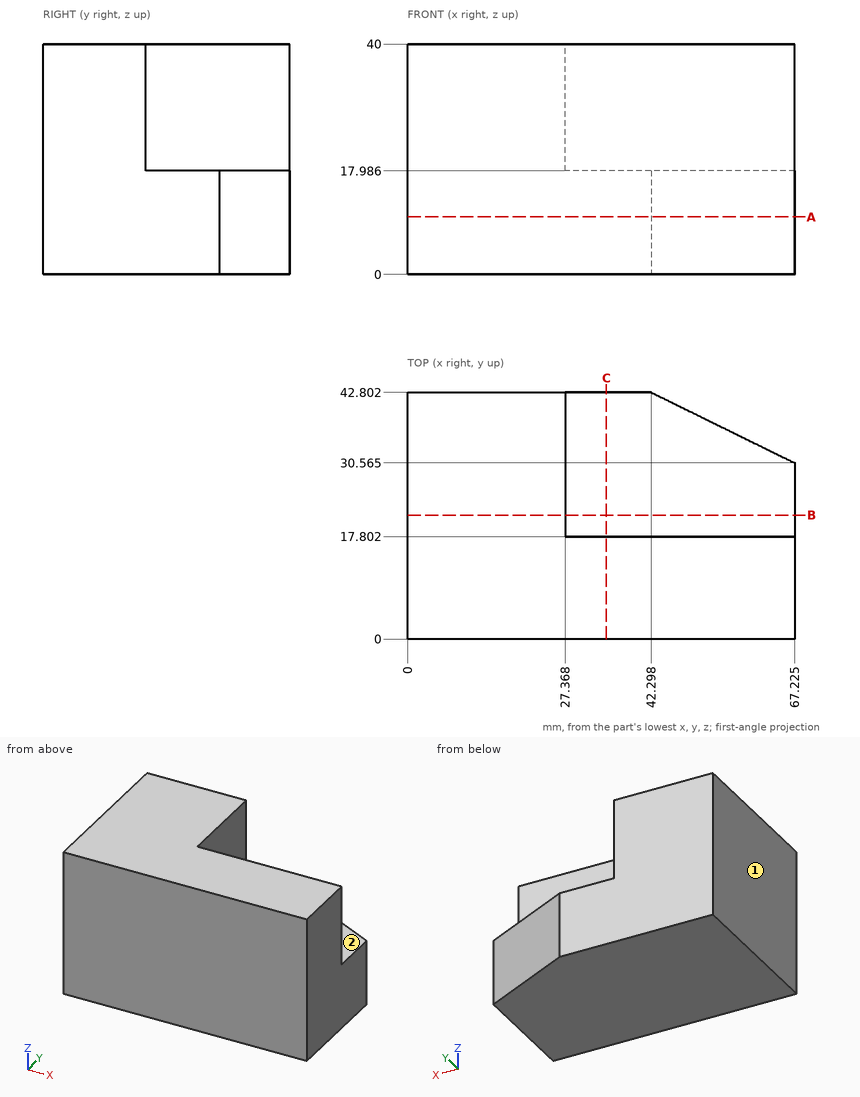
Geometry check sheet. Reference: drawing and pictorial views, mm from the part's lowest x, y, z. A direction names the side the tool comes from. Coordinates: 2 decimals unless noted, no trailing zeros. Order: outer loops, then holes, each group sorted by start corner. A loop starts at its lowest first (then second) coordinate and runs counter-clockwise, first axis right, second up.
1. Go/stop test with a flat-tipped pin: pin 1 Ø17.5 at (x, z) = (38.5, 34) entering from +Y. Record where the tip stops, or that it passes through.
Results found:
pin 1: stops at y = 17.8
2. Sectioned sample at A-A, the plane z = 10. Record the cut outline in (x, y) (1 decimal), and give its area (4 significant figures).
Results found:
outline: (0, 0) - (67.2, 0) - (67.2, 30.6) - (42.3, 42.8) - (0, 42.8) - close
area: 2,725 mm2
3. Scan lines: line 1 (Y direction, x = 62, z = 34); line 2 (X direction, y = 21, z = 18.5); line 3 (Z direction, x = 30.5, y = 18). Record each from-to range of solid material in increasing order.
Results found:
line 1: y = 0 to 17.8
line 2: x = 0 to 27.37
line 3: z = 0 to 17.99
4. Sectioned sample at C-C, the plane x = 34.5. Record the cut outline in (y, z).
Results found:
outline: (0, 0) - (42.8, 0) - (42.8, 17.99) - (17.8, 17.99) - (17.8, 40) - (0, 40) - close
5. Sectioned sample at B-B, the plane y = 21.5. Record the cut outline in (x, z) (1 decimal), and give its area (3 significant figures).
Results found:
outline: (0, 0) - (67.2, 0) - (67.2, 18) - (27.4, 18) - (27.4, 40) - (0, 40) - close
area: 1,810 mm2
6. Set-up check for the marked faces 1 and 2: record each of +Z, -Z, +X, -X, +Y, -Y from which the full face is reachable in a straight line by a thin tool's end or side.
Results found:
face 1: +Z, -Z, -X, +Y, -Y
face 2: +Z, +X, +Y
